```python
from build123d import *

# Parameters (mm, degrees)
SKETCH1_R              = 14.2
SKETCH1_R_2            = 1.65
BASE_DEPTH             = 3.175
SKETCH3_R              = 1.65
STRUT_HOLES_DEPTH      = 4.175
LIGHTENING_HOLES_DEPTH = 4.175


with BuildPart() as part:
    # Sketch1 → Base (new body)
    with BuildSketch(Plane.XY):
        with BuildLine():
            Line((-113.35576806, -30.824729171), (-235.437134887, -94.376266227))
            ThreePointArc((-235.437134887, -94.376266227), (-237.896976574, -97.307791395), (-237.563445987, -101.120063459))
            Line((-237.563445987, -101.120063459), (-219.093501457, -136.600496786))
            ThreePointArc((-219.093501457, -136.600496786), (-216.161976289, -139.060338474), (-212.349704225, -138.726807886))
            Line((-212.349704225, -138.726807886), (-101.120845899, -80.824729171))
            ThreePointArc((-101.120845899, -80.824729171), (-95.519277876, -78.716448255), (-89.577130568, -78))
            Line((-89.577130568, -78), (89.577130568, -78))
            ThreePointArc((89.577130568, -78), (95.519277876, -78.716448255), (101.120845899, -80.824729171))
            Line((101.120845899, -80.824729171), (212.349704225, -138.726807886))
            ThreePointArc((212.349704225, -138.726807886), (216.161976289, -139.060338474), (219.093501457, -136.600496786))
            Line((219.093501457, -136.600496786), (237.563445987, -101.120063459))
            ThreePointArc((237.563445987, -101.120063459), (237.896976574, -97.307791395), (235.437134887, -94.376266227))
            Line((235.437134887, -94.376266227), (113.35576806, -30.824729171))
            ThreePointArc((113.35576806, -30.824729171), (107.754200038, -28.716448255), (101.812052729, -28))
            Line((101.812052729, -28), (-101.812052729, -28))
            ThreePointArc((-101.812052729, -28), (-107.754200038, -28.716448255), (-113.35576806, -30.824729171))
        make_face()
        with Locations((-200, -104.11341011)):
            Circle(SKETCH1_R, mode=Mode.SUBTRACT)
        with Locations((-216.690046638, -98.851058619)):
            Circle(SKETCH1_R_2, mode=Mode.SUBTRACT)
        with Locations((-194.737648509, -87.423363472)):
            Circle(SKETCH1_R_2, mode=Mode.SUBTRACT)
        with Locations((-183.309953362, -109.375761602)):
            Circle(SKETCH1_R_2, mode=Mode.SUBTRACT)
        with Locations((-205.262351491, -120.803456748)):
            Circle(SKETCH1_R_2, mode=Mode.SUBTRACT)
        with Locations((205.262351491, -120.803456748)):
            Circle(SKETCH1_R_2, mode=Mode.SUBTRACT)
        with Locations((216.690046638, -98.851058619)):
            Circle(SKETCH1_R_2, mode=Mode.SUBTRACT)
        with Locations((194.737648509, -87.423363472)):
            Circle(SKETCH1_R_2, mode=Mode.SUBTRACT)
        with Locations((183.309953362, -109.375761602)):
            Circle(SKETCH1_R_2, mode=Mode.SUBTRACT)
        with Locations((200, -104.11341011)):
            Circle(SKETCH1_R, mode=Mode.SUBTRACT)
        with Locations((-10, -47.226497308)):
            Circle(SKETCH1_R_2, mode=Mode.SUBTRACT)
        with Locations((10, -47.226497308)):
            Circle(SKETCH1_R_2, mode=Mode.SUBTRACT)
        with Locations((0, -64.547005384)):
            Circle(SKETCH1_R_2, mode=Mode.SUBTRACT)
    extrude(amount=BASE_DEPTH)

    # Sketch3 → Strut Holes (cut, through all)
    with BuildSketch(Plane.XY.offset(3.175)):
        with Locations((-214.658447291, -134.29175372)):
            Circle(SKETCH3_R)
        with Locations((-148.132634803, -99.660607727)):
            Circle(SKETCH3_R)
        with Locations((-78.03119405, -73)):
            Circle(SKETCH3_R)
        with Locations((-78.03119405, -33)):
            Circle(SKETCH3_R)
        with Locations((-166.602579332, -64.1801744)):
            Circle(SKETCH3_R)
        with Locations((-233.128391821, -98.811320393)):
            Circle(SKETCH3_R)
        with Locations((233.128391821, -98.811320393)):
            Circle(SKETCH3_R)
        with Locations((166.602579332, -64.1801744)):
            Circle(SKETCH3_R)
        with Locations((78.03119405, -33)):
            Circle(SKETCH3_R)
        with Locations((78.03119405, -73)):
            Circle(SKETCH3_R)
        with Locations((148.132634803, -99.660607727)):
            Circle(SKETCH3_R)
        with Locations((214.658447291, -134.29175372)):
            Circle(SKETCH3_R)
    extrude(amount=-STRUT_HOLES_DEPTH, mode=Mode.SUBTRACT)

    # Sketch4 → Lightening Holes (cut, through all)
    with BuildSketch(Plane(origin=(0, 0, 0), x_dir=(-1, 0, 0), z_dir=(0, 0, -1))):
        with BuildLine():
            Line((-168.960154528, -104.865818506), (-160.358460468, -100.38806))
            ThreePointArc((-160.358460468, -100.38806), (-158.749015825, -99.059097441), (-157.82234729, -97.188873132))
            ThreePointArc((-157.82234729, -97.188873132), (-152.750120935, -90.790499395), (-144.599570492, -90.305531214))
            ThreePointArc((-144.599570492, -90.305531214), (-142.53605719, -90.619165384), (-140.52429527, -90.063047123))
            Line((-140.52429527, -90.063047123), (-105.738332031, -71.954620839))
            ThreePointArc((-105.738332031, -71.954620839), (-98.269905543, -69.096671797), (-90.347714306, -68.008483875))
            ThreePointArc((-90.347714306, -68.008483875), (-88.493641512, -67.607748759), (-86.922263791, -66.545229763))
            Line((-86.922263791, -66.545229763), (-79.009491694, -58.632457666))
            ThreePointArc((-79.009491694, -58.632457666), (-77.556385787, -54.760066484), (-79.516892411, -51.11817906))
            Line((-79.516892411, -51.11817906), (-92.727653164, -41.063765898))
            ThreePointArc((-92.727653164, -41.063765898), (-100.534196684, -38.054529652), (-108.738281928, -39.694837502))
            Line((-108.738281928, -39.694837502), (-154.376753667, -63.452722127))
            ThreePointArc((-154.376753667, -63.452722127), (-155.986198311, -64.781684686), (-156.912866845, -66.651908996))
            ThreePointArc((-156.912866845, -66.651908996), (-161.9850932, -73.050282732), (-170.135643643, -73.535250914))
            ThreePointArc((-170.135643643, -73.535250914), (-172.199156946, -73.221616743), (-174.210918865, -73.777735004))
            Line((-174.210918865, -73.777735004), (-182.812612925, -78.255493511))
            ThreePointArc((-182.812612925, -78.255493511), (-185.133676574, -80.802456106), (-185.255701497, -84.246213479))
            ThreePointArc((-185.255701497, -84.246213479), (-184.701637381, -85.374945921), (-183.883494983, -86.32975846))
            ThreePointArc((-183.883494983, -86.32975846), (-178.711740004, -93.031443393), (-176.188437881, -101.111825618))
            ThreePointArc((-176.188437881, -101.111825618), (-175.875568439, -102.329666609), (-175.268763073, -103.430943694))
            ThreePointArc((-175.268763073, -103.430943694), (-172.377811561, -105.306244811), (-168.960154528, -104.865818506))
        make_face()
        with BuildLine():
            Line((-68.284399705, -68), (-63.199367137, -68))
            ThreePointArc((-63.199367137, -68), (-61.351608072, -66.765366865), (-61.785153575, -64.585786438))
            Line((-61.785153575, -64.585786438), (-68.424239552, -57.946700461))
            ThreePointArc((-68.424239552, -57.946700461), (-69.838453114, -57.360914023), (-71.252666676, -57.946700461))
            Line((-71.252666676, -57.946700461), (-74.132142401, -60.826176185))
            ThreePointArc((-74.132142401, -60.826176185), (-74.691303243, -62.565648815), (-73.60347304, -64.033658123))
            ThreePointArc((-73.60347304, -64.033658123), (-71.563592326, -65.373065627), (-69.908865429, -67.166666667))
            ThreePointArc((-69.908865429, -67.166666667), (-69.197270634, -67.779513042), (-68.284399705, -68))
        make_face()
        with BuildLine():
            Line((-25.430550415, -40.5), (-13.883545032, -60.5))
            ThreePointArc((-13.883545032, -60.5), (-13.883545032, -65.5), (-18.21367205, -68))
            Line((-18.21367205, -68), (-49.228804389, -68))
            ThreePointArc((-49.228804389, -68), (-51.14222155, -67.619397663), (-52.764338294, -66.535533906))
            Line((-52.764338294, -66.535533906), (-72.764338294, -46.535533906))
            ThreePointArc((-72.764338294, -46.535533906), (-73.848202051, -41.086582838), (-69.228804389, -38))
            Line((-69.228804389, -38), (-29.760677434, -38))
            ThreePointArc((-29.760677434, -38), (-27.260677434, -38.669872981), (-25.430550415, -40.5))
        make_face()
        with BuildLine():
            Line((52.764338294, -66.535533906), (72.764338294, -46.535533906))
            ThreePointArc((72.764338294, -46.535533906), (73.848202051, -41.086582838), (69.228804389, -38))
            Line((69.228804389, -38), (29.760677434, -38))
            ThreePointArc((29.760677434, -38), (27.260677434, -38.669872981), (25.430550415, -40.5))
            Line((25.430550415, -40.5), (13.883545032, -60.5))
            ThreePointArc((13.883545032, -60.5), (13.883545032, -65.5), (18.21367205, -68))
            Line((18.21367205, -68), (49.228804389, -68))
            ThreePointArc((49.228804389, -68), (51.14222155, -67.619397663), (52.764338294, -66.535533906))
        make_face()
        with BuildLine():
            Line((68.284399705, -68), (63.199367137, -68))
            ThreePointArc((63.199367137, -68), (61.351608072, -66.765366865), (61.785153575, -64.585786438))
            Line((61.785153575, -64.585786438), (68.424239552, -57.946700461))
            ThreePointArc((68.424239552, -57.946700461), (69.838453114, -57.360914023), (71.252666676, -57.946700461))
            Line((71.252666676, -57.946700461), (74.132142401, -60.826176185))
            ThreePointArc((74.132142401, -60.826176185), (74.691303243, -62.565648815), (73.60347304, -64.033658123))
            ThreePointArc((73.60347304, -64.033658123), (71.563592326, -65.373065627), (69.908865429, -67.166666667))
            ThreePointArc((69.908865429, -67.166666667), (69.197270634, -67.779513042), (68.284399705, -68))
        make_face()
        with BuildLine():
            Line((154.376753667, -63.452722127), (108.738281928, -39.694837502))
            ThreePointArc((108.738281928, -39.694837502), (100.534196684, -38.054529652), (92.727653164, -41.063765898))
            Line((92.727653164, -41.063765898), (79.516892411, -51.11817906))
            ThreePointArc((79.516892411, -51.11817906), (77.556385787, -54.760066484), (79.009491694, -58.632457666))
            Line((79.009491694, -58.632457666), (86.922263791, -66.545229763))
            ThreePointArc((86.922263791, -66.545229763), (88.493641512, -67.607748759), (90.347714306, -68.008483875))
            ThreePointArc((90.347714306, -68.008483875), (98.269905543, -69.096671797), (105.738332031, -71.954620839))
            Line((105.738332031, -71.954620839), (140.52429527, -90.063047123))
            ThreePointArc((140.52429527, -90.063047123), (142.53605719, -90.619165384), (144.599570492, -90.305531214))
            ThreePointArc((144.599570492, -90.305531214), (152.750120935, -90.790499395), (157.82234729, -97.188873132))
            ThreePointArc((157.82234729, -97.188873132), (158.749015825, -99.059097441), (160.358460468, -100.38806))
            Line((160.358460468, -100.38806), (168.960154528, -104.865818506))
            ThreePointArc((168.960154528, -104.865818506), (172.377811561, -105.306244811), (175.268763073, -103.430943694))
            ThreePointArc((175.268763073, -103.430943694), (175.875568439, -102.329666609), (176.188437881, -101.111825618))
            ThreePointArc((176.188437881, -101.111825618), (178.711740004, -93.031443393), (183.883494983, -86.32975846))
            ThreePointArc((183.883494983, -86.32975846), (184.701637381, -85.374945921), (185.255701497, -84.246213479))
            ThreePointArc((185.255701497, -84.246213479), (185.133676574, -80.802456106), (182.812612925, -78.255493511))
            Line((182.812612925, -78.255493511), (174.210918865, -73.777735004))
            ThreePointArc((174.210918865, -73.777735004), (172.199156946, -73.221616743), (170.135643643, -73.535250914))
            ThreePointArc((170.135643643, -73.535250914), (161.9850932, -73.050282732), (156.912866845, -66.651908996))
            ThreePointArc((156.912866845, -66.651908996), (155.986198311, -64.781684686), (154.376753667, -63.452722127))
        make_face()
    extrude(amount=-LIGHTENING_HOLES_DEPTH, mode=Mode.SUBTRACT)


solid = part.part
```
The listing builds one solid part. Answer for the finished solid, in the listing's coordinates (mm). A direction names the side the tool comes from. Round coordinates to 2 decimals unless told otherwise and drop trailing zeros. Write each loop counter-clockwise with the first axis right and the second up, starting at its lowest first coordinate (ties: lowest second). Pieces come first, ordered by that corner, then holes. Notation, with made-up numbers: (81, 44) -> (90, 44) arc R14 ccw to (90, 60) -> close; hole circle Ø3 at (8.25, 23). An arc over 180 degrees is marked (long way). Answer as a JSON object with one key per item and string values. Group by question number.
Q1. Determine the mould class of faces 3 (the face through (-1, -75, 0)), 4 (the face through (-162.09, -73.104, 1.565)), 5 (the face through (-228.46, -118.61, 1.57)) for opening direction Y: pulls with the +Y half, pulls with the -Y half, needs draft (parallel to the pull), parting line crosses it, or undercut.
Q2. Which of the six approach directions +Z, -Z, +X, -X, +Y, -Y give full straight-line access (tool end or side, diameter ignored) to faces 1 (the face through (-152.65, -90.74, 1.57)), 2 (the face through (175.251, -63.045, 1.565))?
Q3. Each of these flat-tipped pins is pushed along its axis until it touches: pin 1 Ø2 at (x, y) = (-78.03, -33) entering from -Z; pin 2 Ø1 at (x, z) = (-52.5, 1.5) entering from -Y. Where does it stop, or does it pass through?
Q4. Section A-A (x = 38.5) is taken. Write down the section's boundary in (y, z) (3 decimals).
Q5. Straight lines are drawn through the part: line 1 along X through (y, z) = (-73, 2.1); line 2 along X through (y, z) = (-80, 0.4); line 3 along Y through (x, z) = (67, 1.65). For each, find the intervals that lie inside material, in ascending order.
Q6. Section B-B (z = 1.1) is taken. Count the separate pieces of the cut face and the enclosed holes in it, plus the area to 3 significant figures.
Check values:
{
 "1": {"face 3": "needs draft", "face 4": "undercut", "face 5": "pulls with the -Y half"},
 "2": {"face 1": "+Z, -Z", "face 2": "+Z, -Z, +X, +Y"},
 "3": {"pin 1": "through", "pin 2": "y = -78"},
 "4": {"outline": "(-78, 0) -> (-68, 0) -> (-68, 3.175) -> (-78, 3.175) -> close; (-38, 0) -> (-28, 0) -> (-28, 3.175) -> (-38, 3.175) -> close"},
 "5": {"line 1": "-194.37 to -161.89, -107.75 to -79.68, -76.38 to 76.38, 79.68 to 107.75, 161.89 to 194.37", "line 2": "-207.82 to -184.72, -121.19 to -99.38, 99.38 to 121.19, 184.72 to 207.82", "line 3": "-78 to -68, -59.37 to -52.3, -38 to -28"},
 "6": {"separate pieces": "1", "enclosed holes": "31", "area": "13,900 mm^2"}
}
